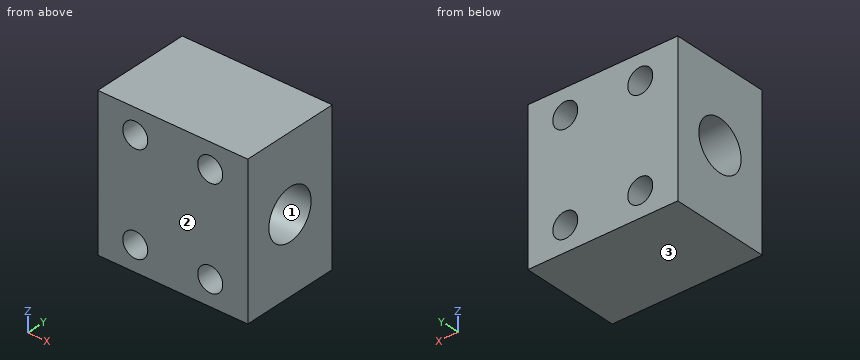
```python
from build123d import *

# Parameters (mm, degrees)
SKETCH1_W           = 38.1
SKETCH1_H           = 38.1
SKETCH1_R           = 3.175
BOSS_EXTRUDE1_DEPTH = 25.4
SKETCH2_R           = 6.35
CUT_EXTRUDE1_DEPTH  = 50.595085442


with BuildPart() as part:
    # Sketch1 → Boss-Extrude1 (new body)
    with BuildSketch(Plane(origin=(0, 0, 0), x_dir=(1, 0, 0), z_dir=(0, 1, 0))):
        Rectangle(SKETCH1_W, SKETCH1_H)
        with Locations(Location((-9.525, 12.7, 0), (0, 0, 270))):
            Circle(SKETCH1_R, mode=Mode.SUBTRACT)
        with Locations(Location((9.525, 12.7, 0), (0, 0, 90))):
            Circle(SKETCH1_R, mode=Mode.SUBTRACT)
        with Locations(Location((9.525, -12.7, 0), (0, 0, 270))):
            Circle(SKETCH1_R, mode=Mode.SUBTRACT)
        with Locations(Location((-9.525, -12.7, 0), (0, 0, 90))):
            Circle(SKETCH1_R, mode=Mode.SUBTRACT)
    extrude(amount=BOSS_EXTRUDE1_DEPTH)

    # Sketch2 → Cut-Extrude1 (cut, through all)
    with BuildSketch(Plane(origin=(19.05, 0, 0), x_dir=(0, 0, -1), z_dir=(1, 0, 0))):
        with Locations((0, 12.7)):
            Circle(SKETCH2_R)
    extrude(amount=-CUT_EXTRUDE1_DEPTH, mode=Mode.SUBTRACT)


solid = part.part
```
Geometry check sheet. Reference: the model listing, model coordinates, mm. Face numbers are marked on the shaded views. Round coordinates to 2 decimals unless told otherwise and drop trailing zeros. Loops run counter-clockwise (first coordinate to the right, second up) from the corner with the lowest first, then second, coordinate; pieces in that order, holes last. Notation, with made-up numbers: (-40, -20.5) - (-12, -20.5) arc R27 ccw to (-12, -3.5) - close; hole circle Ø9 at (-7.75, 57). An arc over 180 degrees is marked (long way). Use a Markdown table: item, result.
Q1. Cross-section at A-A on y = 12.7. Record the cut outline in (x, z) (3 decimals).
Solutions:
| item | result |
|---|---|
| outline | (-19.05, -19.05) - (19.05, -19.05) - (19.05, -6.35) - (-19.05, -6.35) - close; (-19.05, 6.35) - (19.05, 6.35) - (19.05, 19.05) - (-19.05, 19.05) - close; hole circle Ø6.35 at (-9.525, -12.7); hole circle Ø6.35 at (-9.525, 12.7); hole circle Ø6.35 at (9.525, -12.7); hole circle Ø6.35 at (9.525, 12.7) |
Q2. Material ranges on line 1 (X direction, y = 11.5, z = 12.7); line 2 (Z direction, x = 9.5, y = 4); line 3 (Z direction, x = 9, y = 22.5), recorded low to high.
Solutions:
| item | result |
|---|---|
| line 1 | x = -19.05 to -12.7, -6.35 to 6.35, 12.7 to 19.05 |
| line 2 | z = -19.05 to -15.87, -9.53 to 9.53, 15.87 to 19.05 |
| line 3 | z = -19.05 to -15.83, -9.57 to 9.57, 15.83 to 19.05 |
Q3. Cross-section at B-B on z = 0. Record the cut outline in (x, y).
Solutions:
| item | result |
|---|---|
| outline | (-19.05, 0) - (19.05, 0) - (19.05, 6.35) - (-19.05, 6.35) - close; (-19.05, 19.05) - (19.05, 19.05) - (19.05, 25.4) - (-19.05, 25.4) - close |
Q4. Cross-section at D-D on y = 5.5. Record the cut outline in (x, z) (3 decimals).
Solutions:
| item | result |
|---|---|
| outline | (-19.05, -19.05) - (19.05, -19.05) - (19.05, 19.05) - (-19.05, 19.05) - close; hole circle Ø6.35 at (-9.525, -12.7); hole circle Ø6.35 at (-9.525, 12.7); hole circle Ø6.35 at (9.525, -12.7); hole circle Ø6.35 at (9.525, 12.7) |
Q5. Cross-section at C-C on z = 12.7. Record the cut outline in (x, y).
Solutions:
| item | result |
|---|---|
| outline | (-19.05, 0) - (-12.7, 0) - (-12.7, 25.4) - (-19.05, 25.4) - close; (-6.35, 0) - (6.35, 0) - (6.35, 25.4) - (-6.35, 25.4) - close; (12.7, 0) - (19.05, 0) - (19.05, 25.4) - (12.7, 25.4) - close |
Q6. Draft check along Y on the marked faces 1, 2 and 3. Enter one of: released by +Y, released by -Y, zero draft, split by the parting line, or undercut.
Solutions:
| item | result |
|---|---|
| face 1 | undercut |
| face 2 | released by -Y |
| face 3 | zero draft |
